from build123d import *

# Parameters (mm, degrees)
F1_DEPTH = 12
F3_DEPTH = 4
F4_R     = 1


with BuildPart() as f1:
    # F0 (on Top) → F1 (new body)
    with BuildSketch(Plane.XY):
        with BuildLine():
            Line((-200, 28), (-200, 0))
            Line((-200, 0), (200, 0))
            Line((200, 0), (200, 28))
            Line((200, 28), (120, 28))
            ThreePointArc((120, 28), (115.050253, 30.050253), (113, 35))
            Line((113, 35), (113, 50))
            Line((113, 50), (-113, 50))
            Line((-113, 50), (-113, 35))
            ThreePointArc((-113, 35), (-115.050253, 30.050253), (-120, 28))
            Line((-120, 28), (-200, 28))
        make_face()
    extrude(amount=F1_DEPTH)

    # F2 (on face) → F3 (cut)
    with BuildSketch(Plane(origin=(0, 0, 0), x_dir=(1, 0, 0), z_dir=(0, 0, -1))):
        with BuildLine():
            Line((-96.5, -21.899495), (-96.5, -50))
            Line((-96.5, -50), (96.5, -50))
            Line((96.5, -50), (96.5, -21.899495))
            ThreePointArc((96.5, -21.899495), (96.5, -12), (86.600505, -12))
            Line((86.600505, -12), (-86.600505, -12))
            ThreePointArc((-86.600505, -12), (-96.5, -12), (-96.5, -21.899495))
        make_face()
    extrude(amount=-F3_DEPTH, mode=Mode.SUBTRACT)

    # F4
    f4_edges = [f1.edges().sort_by_distance(p)[0] for p in [
        (-200, 0, 6),
        (-200, 28, 6),
        (-113, 50, 6),
        (-96.5, 21.899495, 2),
        (-86.600505, 12, 2),
        (86.600505, 12, 2),
        (96.5, 21.899495, 2),
        (113, 50, 6),
        (200, 28, 6),
        (200, 0, 6),
    ]]
    fillet(f4_edges, radius=F4_R)


solid = f1.part
Model file for the job. Use its own axes, mm. A direction names the side the tool comes from. Give positions to 0.01 mm unless a question says otherwise; leave off trailing zeros. Write each loop counter-clockwise with the first axis right and the second up, starting at its lowest first coordinate (ties: lowest second). Pieces come first, ordered by that corner, then holes. Notation, with made-up numbers: M -25,37 L 24,37 A23 ccw 24,73 Z; hole C 25,73.5 d10. An arc over 180 degrees is marked long. One line per item, written item: value. Start each with the question number.
Q1. Saw through at D-D, the plane x = -132.5. Write the cut outline in (y, z).
Q2. Two-plate mould, pull along Y, no slides. Class faces 4 (the flat face through (-200, 14, 6)), 5 (the cylindrical face through (-96.4, 11.9, 2)), 6 (the cylindrical face through (96.6, 12.1, 2)), 7 (the flat face through (2, 50, 7)): +Y half, -Y half, draft (parallel to the pull), parting line (faces both ways), or undercut.
Q3. Drop flat-ended pins along their axis: pin 1 Ø6 at (x, z) = (170.5, 6) entering from +Y; pin 2 Ø4.5 at (x, z) = (-37, 1) entering from +Y; pin 3 Ø4.5 at (y, z) = (33.5, 1.5) entering from -X. Give the stop position or say it passes through.
Q4. Saw through at B-B, the plane z = 8. Write the cut outline in (x, y), plus the area to 3 significant figures.
Q5. Probe probe 1 along X at (y, z) = (45, 2.75); probe 2 along X at (y, z) = (27, 3.75); probe 3 along X at (y, z) = (10.5, 3.75). List the from-to ranges inside material, lowest first. Write a range as [from, to].
Q6. Saw through at C-C, the plane x = -22. Write the cut outline in (y, z).
Q7. 3-axis set-ups, long thin cutter, end or side, ignore diameter. For faces 1 (the flat face through (113, 42, 6)), 2 (the flat face through (-159, 28, 6)), 3 (the flat face through (-3, 20, 12)): which of +Z, -Z, +X, -X, +Y, -Y reach the whole face in a straight line?
Q8. Saw through at A-A, the plane y = 41.5. Write the cut outline in (x, z).
Output values:
1. outline: M 0,0 L 28,0 L 28,12 L 0,12 Z
2. face 4: draft
2. face 5: undercut
2. face 6: undercut
2. face 7: +Y half
3. pin 1: stops at y = 28
3. pin 2: stops at y = 12
3. pin 3: stops at x = -114.09
4. outline: M -200,1 A1 ccw -199,0 L 199,0 A1 ccw 200,1 L 200,27 A1 ccw 199,28 L 120,28 A7 cw 113,35 L 113,49 A1 ccw 112,50 L -112,50 A1 ccw -113,49 L -113,35 A7 cw -120,28 L -199,28 A1 ccw -200,27 Z
4. area: 16,200 mm²
5. probe 1: x = [-113, -96.5], [96.5, 113]
5. probe 2: x = [-200, -96.5], [96.5, 200]
5. probe 3: x = [-200, -94.27], [-88.83, 88.83], [94.27, 200]
6. outline: M 0,0 L 12,0 L 12,4 L 50,4 L 50,12 L 0,12 Z
7. face 1: +Z, -Z, +X, +Y
7. face 2: +Z, -Z, -X, +Y
7. face 3: +Z, +X, -X, +Y, -Y
8. outline: M -113,0 L -96.5,0 L -96.5,4 L 96.5,4 L 96.5,0 L 113,0 L 113,12 L -113,12 Z
